Build history of the part. All positions in model axes, mm. Face numbers are marked on the shaded views. A direction names the side the tool comes from. Round coordinates to 2 decimals unless told otherwise and drop trailing zeros. Loops run counter-clockwise (first coordinate to the right, second up) from the corner with the lowest first, then second, coordinate; pieces in that order, holes last. Notation, with made-up numbers: (54.25, 1) - (80.25, 1) arc R26 ccw to (80.25, 23) - close; hole circle Ø3 at (-0.5, -25.75). An arc over 180 degrees is marked (long way). Use a Markdown table: item, result.
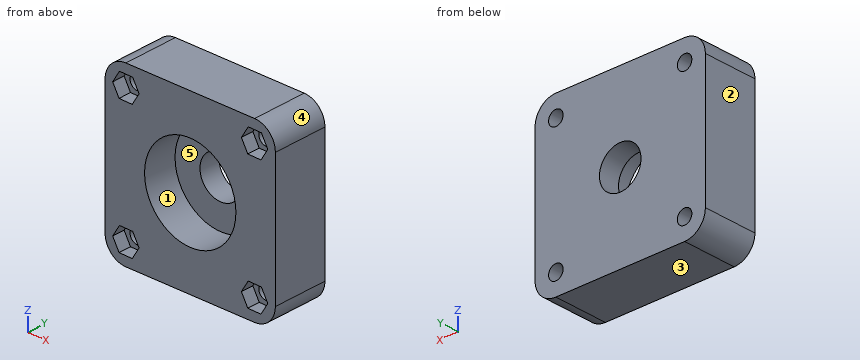
from build123d import *

# Parameters (mm, degrees)
SKETCH1_R           = 11
SKETCH1_R_2         = 1.75
BOSS_EXTRUDE1_DEPTH = 8
SKETCH2_R           = 1.75
SKETCH2_R_2         = 5
BOSS_EXTRUDE2_DEPTH = 5
CUT_EXTRUDE1_DEPTH  = 3


with BuildPart() as part:
    # Sketch1 → Boss-Extrude1 (new body)
    with BuildSketch(Plane(origin=(0, 0, 0), x_dir=(1, 0, 0), z_dir=(0, 1, 0))):
        with BuildLine():
            Line((-15.5, 20.5), (15.5, 20.5))
            ThreePointArc((15.5, 20.5), (19.035533906, 19.035533906), (20.5, 15.5))
            Line((20.5, 15.5), (20.5, -15.5))
            ThreePointArc((20.5, -15.5), (19.035533906, -19.035533906), (15.5, -20.5))
            Line((15.5, -20.5), (-15.5, -20.5))
            ThreePointArc((-15.5, -20.5), (-19.035533906, -19.035533906), (-20.5, -15.5))
            Line((-20.5, -15.5), (-20.5, 15.5))
            ThreePointArc((-20.5, 15.5), (-19.035533906, 19.035533906), (-15.5, 20.5))
        make_face()
        Circle(SKETCH1_R, mode=Mode.SUBTRACT)
        with Locations((-15.5, 15.5)):
            Circle(SKETCH1_R_2, mode=Mode.SUBTRACT)
        with Locations((15.5, 15.5)):
            Circle(SKETCH1_R_2, mode=Mode.SUBTRACT)
        with Locations((15.5, -15.5)):
            Circle(SKETCH1_R_2, mode=Mode.SUBTRACT)
        with Locations((-15.5, -15.5)):
            Circle(SKETCH1_R_2, mode=Mode.SUBTRACT)
    extrude(amount=BOSS_EXTRUDE1_DEPTH)

    # Sketch2 → Boss-Extrude2 (add)
    with BuildSketch(Plane(origin=(0, 8, 0), x_dir=(1, 0, 0), z_dir=(0, 1, 0))):
        with BuildLine():
            Line((-20.5, 15.5), (-20.5, -15.5))
            ThreePointArc((-20.5, -15.5), (-19.035533906, -19.035533906), (-15.5, -20.5))
            Line((-15.5, -20.5), (15.5, -20.5))
            ThreePointArc((15.5, -20.5), (19.035533906, -19.035533906), (20.5, -15.5))
            Line((20.5, -15.5), (20.5, 15.5))
            ThreePointArc((20.5, 15.5), (19.035533906, 19.035533906), (15.5, 20.5))
            Line((15.5, 20.5), (-15.5, 20.5))
            ThreePointArc((-15.5, 20.5), (-19.035533906, 19.035533906), (-20.5, 15.5))
        make_face()
        with Locations((15.5, 15.5)):
            Circle(SKETCH2_R, mode=Mode.SUBTRACT)
        with Locations((15.5, -15.5)):
            Circle(SKETCH2_R, mode=Mode.SUBTRACT)
        with Locations((-15.5, 15.5)):
            Circle(SKETCH2_R, mode=Mode.SUBTRACT)
        Circle(SKETCH2_R_2, mode=Mode.SUBTRACT)
        with Locations((-15.5, -15.5)):
            Circle(SKETCH2_R, mode=Mode.SUBTRACT)
    extrude(amount=BOSS_EXTRUDE2_DEPTH)

    # Sketch3 → Cut-Extrude1 (cut)
    with BuildSketch(Plane.XZ):
        Polygon((-13.860691665, 18.219559066), (-17.035553071, 18.279462196), (-18.674861406, 15.55990313), (-17.139308335, 12.780440934), (-13.964446929, 12.720537804), (-12.325138594, 15.44009687), align=None)
        Polygon((12.325138594, 15.55990313), (13.860691665, 12.780440934), (17.035553071, 12.720537804), (18.674861406, 15.44009687), (17.139308335, 18.219559066), (13.964446929, 18.279462196), align=None)
        Polygon((13.964446929, -12.720537804), (12.325138594, -15.44009687), (13.860691665, -18.219559066), (17.035553071, -18.279462196), (18.674861406, -15.55990313), (17.139308335, -12.780440934), align=None)
        Polygon((-13.860691665, -12.780440934), (-17.035553071, -12.720537804), (-18.674861406, -15.44009687), (-17.139308335, -18.219559066), (-13.964446929, -18.279462196), (-12.325138594, -15.55990313), align=None)
    extrude(amount=-CUT_EXTRUDE1_DEPTH, mode=Mode.SUBTRACT)


solid = part.part
Q1. Which spindle directions (+Z, -Z, +X, -X, +Y, -Y) get a long thin tool onto all of the face, cutting with end or side? Do the marked faces 4 and 5. Say none if no direction does.
Results found:
| item | result |
|---|---|
| face 4 | +Z, +X, +Y, -Y |
| face 5 | -Y |
Q2. Drop flat-ended pins along their axis: pin 1 (6 mm diameter, centred on x = 17, z = 15, fed in from -Y); pin 2 (8 mm diameter, centred on x = 0, z = 0, fed in from +Y); pin 3 (4 mm diameter, centred on x = 15.5, z = -15.5, fed in from -Y); pin 4 (10 mm diameter, centred on x = 1.5, z = 2.5, fed in from -Y). Give the stop position or say it passes through.
Results found:
| item | result |
|---|---|
| pin 1 | stops at y = 0 |
| pin 2 | passes through |
| pin 3 | stops at y = 3 |
| pin 4 | stops at y = 8 |
Q3. Cut at B-B, the plane x = 0. List the corners of the cut face in (y, z).
Results found:
| item | result |
|---|---|
| outline | (0, -20.5) - (13, -20.5) - (13, -5) - (8, -5) - (8, -11) - (0, -11) - close; (0, 11) - (8, 11) - (8, 5) - (13, 5) - (13, 20.5) - (0, 20.5) - close |
Q4. Cut at D-D, the plane x = -16.5. List the corners of the cut face in (y, z), plus the area to 3 significant figures.
Results found:
| item | result |
|---|---|
| outline | (0, -20.4) - (13, -20.4) - (13, -16.94) - (3, -16.94) - (3, -18.23) - (0, -18.23) - close; (0, -12.73) - (3, -12.73) - (3, -14.06) - (13, -14.06) - (13, 14.06) - (3, 14.06) - (3, 12.77) - (0, 12.77) - close; (0, 18.27) - (3, 18.27) - (3, 16.94) - (13, 16.94) - (13, 20.4) - (0, 20.4) - close |
| area | 440 mm2 |
Q5. Probe line 1 (Z direction, x = 15.5, y = 7); line 2 (Z direction, x = 0, y = 9.7). List the from-to ranges inside material, lowest first.
Results found:
| item | result |
|---|---|
| line 1 | z = -20.5 to -17.25, -13.75 to 13.75, 17.25 to 20.5 |
| line 2 | z = -20.5 to -5, 5 to 20.5 |
Q6. Cut at A-A, the plane z = 0. List the corners of the cut face in (x, y), plus the area to 3 significant figures.
Results found:
| item | result |
|---|---|
| outline | (-20.5, 0) - (-11, 0) - (-11, 8) - (-5, 8) - (-5, 13) - (-20.5, 13) - close; (5, 8) - (11, 8) - (11, 0) - (20.5, 0) - (20.5, 13) - (5, 13) - close |
| area | 307 mm2 |
Q7. Pull direction X, two halves, no side cores. Call the marked faces 1, 2 and 3: pulls with the +X half, pulls with the -X half, needs draft (parallel to the pull), parting line crosses it, or undercut.
Results found:
| item | result |
|---|---|
| face 1 | undercut |
| face 2 | pulls with the -X half |
| face 3 | needs draft |
Q8. Cut at C-C, the plane y = 9.5. List the corners of the cut face in (x, z), plus the area to 3 significant figures.
Results found:
| item | result |
|---|---|
| outline | (-20.5, -15.5) arc R5 ccw to (-15.5, -20.5) - (15.5, -20.5) arc R5 ccw to (20.5, -15.5) - (20.5, 15.5) arc R5 ccw to (15.5, 20.5) - (-15.5, 20.5) arc R5 ccw to (-20.5, 15.5) - close; hole circle Ø3.5 at (-15.5, -15.5); hole circle Ø3.5 at (-15.5, 15.5); hole circle Ø10 at (0, 0); hole circle Ø3.5 at (15.5, -15.5); hole circle Ø3.5 at (15.5, 15.5) |
| area | 1,540 mm2 |
